Input: part model. Units: mm. Frame: model coordinates. A direction names the side the tool comes from. Coordinates: 2 decimals unless noted, no trailing zeros. Write each loop counter-clockwise with the first axis right and the second up, starting at its lowest first coordinate (ties: lowest second). Pieces come first, ordered by that corner, then holes. Notation, with made-up numbers: M 62.25,42.5 L 96.25,42.5 A19 ccw 96.25,76.5 Z; hole C 28,33.5 d3. An arc over 180 degrees is marked long. Answer as a JSON object with one key per item and string values. Group by question number.
from build123d import *

# Parameters (mm, degrees)
F1_DEPTH = 1.27
F0_W     = 7.62
F0_H     = 5.08
F2_DEPTH = 7.62
F3_DEPTH = 1.27
F4_DEPTH = 25.4
F5_R     = 25.39999
F6_R     = 25.39999


# Not quite as in the source:
# - a fillet or chamfer is up to 0.001 mm smaller than in the source, because OpenCascade refuses the exact size


with BuildPart() as f1:
    # F0 (on Top) → F1 (new body)
    with BuildSketch(Plane.XY):
        Polygon((-56.5321096511, 32.319452062), (-145.4321096511, 32.319452062), (-145.4321096511, 23.429452062), (-130.9795096511, 23.429452062), (-130.9795096511, 28.509452062), (-123.3595096511, 28.509452062), (-123.3595096511, 23.429452062), (-108.9069096511, 23.429452062), (-108.9069096511, 28.509452062), (-101.2869096511, 28.509452062), (-101.2869096511, 23.429452062), (-56.5321096511, 23.429452062), align=None)
    extrude(amount=F1_DEPTH)



with BuildPart() as f2:
    # F0 (on Top) → F2 (new body)
    with BuildSketch(Plane.XY):
        with Locations((-127.1695096511, 25.969452062)):
            Rectangle(F0_W, F0_H)
    extrude(amount=-F2_DEPTH)


with BuildPart() as f2b:
    # F0 (on Top) → F2, piece 2 (new body)
    with BuildSketch(Plane.XY):
        with Locations((-105.0969096511, 25.969452062)):
            Rectangle(F0_W, F0_H)
    extrude(amount=-F2_DEPTH)


with BuildPart() as f1_1:
    add(f1.part)

    add(f2.part)  # F3 merges F2

    add(f2b.part)  # F3 merges F2b
    # F0 (on Top) → F3 (join)
    with BuildSketch(Plane.XY):
        with Locations((-127.1695096511, 25.969452062)):
            Rectangle(F0_W, F0_H)
        with Locations((-105.0969096511, 25.969452062)):
            Rectangle(F0_W, F0_H)
    extrude(amount=F3_DEPTH)

    # F0 (on Top) → F4 (join)
    with BuildSketch(Plane.XY):
        Polygon((-31.1321096511, 32.319452062), (-56.5321096511, 32.319452062), (-56.5321096511, 23.429452062), (-56.5321096511, -5.780547938), (-31.1321096511, -5.780547938), align=None)
    extrude(amount=F4_DEPTH)

    # F5 (radius 25.4 in the source; OpenCascade refuses exactly that, so slightly less here)
    f5_edges = [f1_1.edges().sort_by_distance(p)[0] for p in [
        (-31.13211, 13.269452, 0),
    ]]
    fillet(f5_edges, radius=F5_R)

    # F6 (radius 25.4 in the source; OpenCascade refuses exactly that, so slightly less here)
    f6_edges = [f1_1.edges().sort_by_distance(p)[0] for p in [
        (-56.53211, 13.269452, 25.4),
    ]]
    fillet(f6_edges, radius=F6_R)


solid = f1_1.part
Q1. Section C-C, the plane z = 7.5. Return the cut outline in (x, y), and give its area (3 significant figures).
Q2. Section D-D, the plane x = -88. Return the cut outline in (y, z).
Q3. Line query: line 1 (X direction, y = 25, z = -1); line 2 (Z direction, x = -59.5, y = 25.5); line 3 (X direction, y = 8, z = 4). Output: solid intervals per line, ascending. Write a range as from..to.
Q4. Pin query (flat end, axial travel): pin 1 Ø4 at (y, z) = (26, -4) entering from +X; pin 2 Ø6 at (x, z) = (-102.5, 3.5) entering from -Y; pin 3 Ø1.5 at (y, z) = (27, -3) entering from -X; pin 4 Ø6 at (x, y) = (-60.5, 10.5) entering from +Z. Return the tip coordinate at first contact, or that it passes through.
Q5. Draft query along X for faces 4 (the flat face through (-123.36, 26, -4)), 5 (the flat face through (-101.287, 26, -4)), 6 (the flat face through (-108.907, 26, -4)), 7 (the flat face through (-105, 26, -7.62)). Return one class per face: released by +X, released by -X, zero draft, split by the parting line, or undercut.
Q6. Section B-B, the plane x = -127. Return the cut outline in (y, z).
Q7. Access query for faces 1 (the flat face through (-105, 28.509, -4)), 2 (the flat face through (-130.98, 26, -4)), 3 (the flat face through (-108, 23.429, -2)). Directions: +Z, -Z, +X, -X, +Y, -Y. A direction counts if a zero-diameter tool reaches every point of the face in a straight line with its end or side. Return the directions, or none.
Filled in:
{
 "1": {"outline": "M -55.4,-5.78 L -38.51,-5.78 L -38.51,32.32 L -55.4,32.32 Z", "area": "643 mm^2"},
 "2": {"outline": "M 23.43,0 L 32.32,0 L 32.32,1.27 L 23.43,1.27 Z"},
 "3": {"line 1": "-130.98..-123.36, -108.91..-101.29", "line 2": "0..1.27", "line 3": "-56.22..-42.85"},
 "4": {"pin 1": "x = -101.29", "pin 2": "y = 23.43", "pin 3": "x = -130.98", "pin 4": "through"},
 "5": {"face 4": "undercut", "face 5": "released by +X", "face 6": "undercut", "face 7": "zero draft"},
 "6": {"outline": "M 23.43,-7.62 L 28.51,-7.62 L 28.51,0 L 32.32,0 L 32.32,1.27 L 23.43,1.27 Z"},
 "7": {"face 1": "-Z, +X, -X, +Y", "face 2": "-Z, -X, +Y, -Y", "face 3": "+Z, -Z, -X, -Y"}
}
